from build123d import *

# Parameters (mm, degrees)
CYLINDER018_R     = 6.2
CYLINDER018_DEPTH = 5
TUBE_R            = 7
TUBE_R_2          = 3
TUBE_DEPTH        = 7


with BuildPart() as cylinder:
    # Cylinder018 → Cylinder018 (new body)
    with BuildSketch(Plane(origin=(40, 0, 3), x_dir=(1, 0, 0), z_dir=(0, 0, 1))):
        Circle(CYLINDER018_R)
    extrude(amount=CYLINDER018_DEPTH)


with BuildPart() as captmp:
    # Tube → Tube (new body)
    with BuildSketch(Plane(origin=(40, 0, 0), x_dir=(1, 0, 0), z_dir=(0, 0, 1))):
        Circle(TUBE_R)
        Circle(TUBE_R_2, mode=Mode.SUBTRACT)
    extrude(amount=TUBE_DEPTH)

    # Cut011: cut Cylinder
    add(cylinder.part, mode=Mode.SUBTRACT)


solid = captmp.part
Geometry: final body of the model. Coordinates: model frame, mm. A direction names the side the tool comes from. Give positions to 0.01 mm unless a question says otherwise; leave off trailing zeros. Order: outer loops, then holes, each group sorted by start corner. A loop starts at its lowest first (then second) coordinate and runs counter-clockwise, first axis right, second up. Notation, with made-up numbers: (-8, 11) -> (48, 11) arc R24 ccw to (48, 26) -> close; hole circle Ø8 at (48, 36.25). An arc over 180 degrees is marked (long way). Put each result on its own line as item: value.
Q1. Pin query (flat end, axial travel): pin 1 (6 mm diameter, centred on x = 42, y = 1.5, fed in from +Z); pin 2 (2 mm diameter, centred on x = 38.5, z = 4, fed in from -Y); pin 3 (1.5 mm diameter, centred on y = 5, z = 4, fed in from -X); pin 4 (5 mm diameter, centred on x = 40, y = 0, fed in from +Z). Return the tip coordinate at first contact, or that it passes through.
Here are the results:
pin 1: stops at z = 3
pin 2: stops at y = -6.98
pin 3: stops at x = 34.44
pin 4: passes through
Q2. Draft query along Y for faces 1 (the face through (35.1, -3.8, 5)), 2 (the face through (46.677, 2.103, 3.451)), 3 (the face through (36, -5, 7)). Return one class per face: released by +Y, released by -Y, zero draft, split by the parting line, or undercut.
Here are the results:
face 1: undercut
face 2: split by the parting line
face 3: zero draft
Q3. Section C-C, the plane z = 4.25. Return loops of the section in (x, y).
Here are the results:
outline: circle Ø14 at (40, 0); hole circle Ø12.4 at (40, 0)
Q4. Section B-B, the plane x = 41.75. Return loops of the section in (y, z), then the cut area to 3 significant figures.
Here are the results:
outline: (-6.78, 0) -> (-2.44, 0) -> (-2.44, 3) -> (-5.95, 3) -> (-5.95, 7) -> (-6.78, 7) -> close; (2.44, 0) -> (6.78, 0) -> (6.78, 7) -> (5.95, 7) -> (5.95, 3) -> (2.44, 3) -> close
area: 32.7 mm^2
Q5. Section A-A, the plane y = 0. Return loops of the section in (x, z), then the cut area to 3 significant figures.
Here are the results:
outline: (33, 0) -> (37, 0) -> (37, 3) -> (33.8, 3) -> (33.8, 7) -> (33, 7) -> close; (43, 0) -> (47, 0) -> (47, 7) -> (46.2, 7) -> (46.2, 3) -> (43, 3) -> close
area: 30.4 mm^2
Q6. Reachability of faces 4 (the face through (43, 1, 3)), 5 (the face through (41, -3, 0)) from +Z, -Z, +X, -X, +Y, -Y: full face, straight path, thin tool, end or side. Return the list, or none.
Here are the results:
face 4: +Z
face 5: -Z, +X, -X, +Y, -Y
Q7. Section D-D, the plane y = -5.5. Return loops of the section in (x, z).
Here are the results:
outline: (35.67, 0) -> (44.33, 0) -> (44.33, 7) -> (42.86, 7) -> (42.86, 3) -> (37.14, 3) -> (37.14, 7) -> (35.67, 7) -> close
Q8. Material intervals for L1, parallel to Y at x = 40, z = 5.15; L2, parallel to Z at x = 40.5, y = 5.5; L3, parallel to X at y = -4.75, z = 3.75, sorted ascending.
Here are the results:
L1: y = -7 to -6.2, 6.2 to 7
L2: z = 0 to 3
L3: x = 34.86 to 36.02, 43.98 to 45.14
